Can you work these out from the drawing? Everything is in mm from the part's minimum corner. A direction names the side the tool comes from. Give positions to 0.01 mm unless a question says otherwise; leave off trailing zeros. Loops run counter-clockwise (first coordinate to the right, second up) from the corner with the lowest first, then second, coordinate; pieces in that order, holes last. Notation, with made-up numbers: (-12, 76) - (27, 76) arc R22 ccw to (27, 99) - close; hole circle Ø4 at (33, -39). An arc over 180 degrees is marked (long way). Answer in a Markdown table with one row per item.
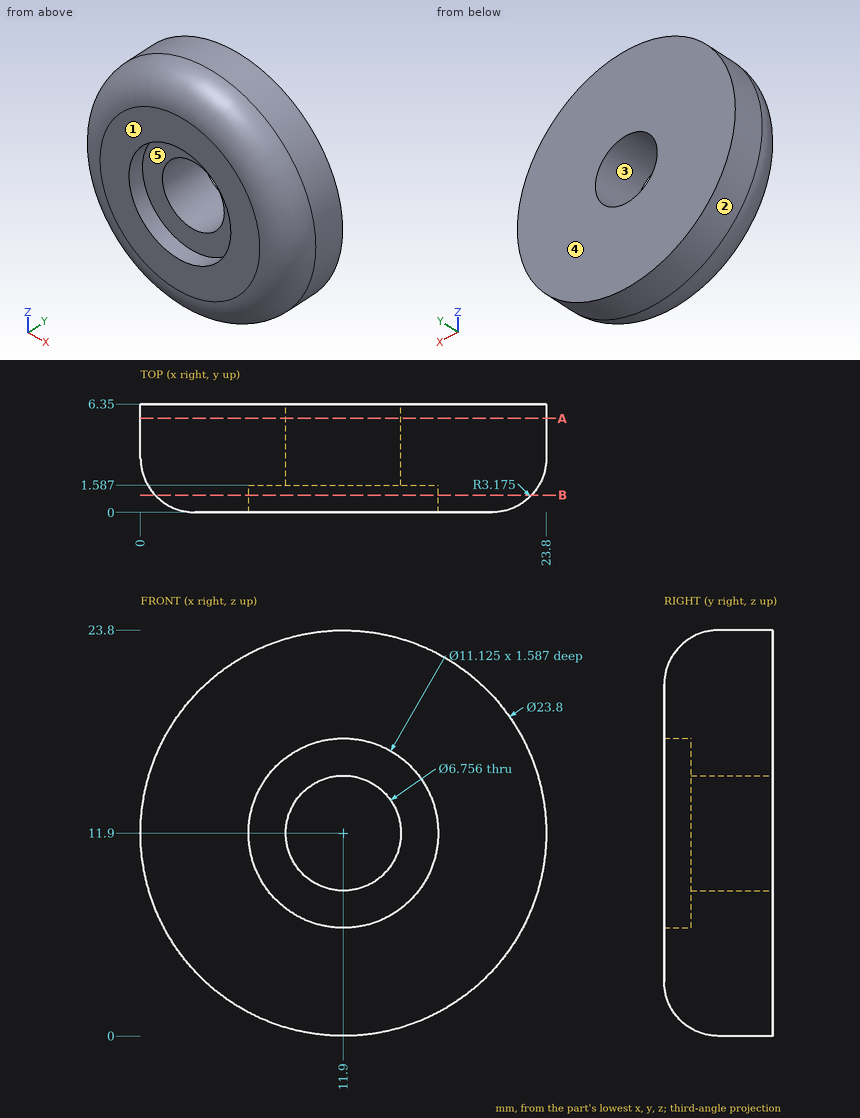
Q1. For pin 1 (1 mm diameter, centred on x = 15, z = 14, fed in from -Y); pin 2 (1.5 mm diameter, centred on y = 1, z = 12.5, fed in from +X); pin 3 (2 mm diameter, centred on y = 3.5, z = 6, fed in from -X) (1 decimal), each with a flat end and sliding along its axis, tell me the tip position at first contact or that it passes through.
Checked values:
| item | result |
|---|---|
| pin 1 | stops at y = 1.59 |
| pin 2 | stops at x = 23.45 |
| pin 3 | stops at x = 1.1 |
Q2. If I drill on line 1 (Z direction, x = 9.25, y = 0.5) (1 decimal); line 2 (Z direction, x = 14.25, y = 4.75) (1 decimal); line 3 (Y direction, x = 9.5, z = 16.5), over which ranges is the centre line in solid material (lowest first)? Write a range as [from, to].
Checked values:
| item | result |
|---|---|
| line 1 | z = [1.8, 7], [16.8, 22] |
| line 2 | z = [0.2, 9.5], [14.3, 23.6] |
| line 3 | y = [1.59, 6.35] |
Q3. On a 3-axis mill with a long thin cutter (end or side, diameter ignored), from which of +Z, -Z, +X, -X, +Y, -Y can I reach the whole of each face in a straight line? I mean the marked faces 4 and 5. Say none if no direction works.
Checked values:
| item | result |
|---|---|
| face 4 | +Z, -Z, +X, -X, +Y |
| face 5 | -Y |
Q4. Imagine slicing it at B-B, the plane y = 1. Write out the boundary of the cut face in (x, z) (1 decimal).
Checked values:
| item | result |
|---|---|
| outline | circle Ø22.1 at (11.9, 11.9); hole circle Ø11.1 at (11.9, 11.9) |
Q5. Imagine slicing it at A-A, the plane y = 5.5. Write out the boundary of the cut face in (x, z), and give its area (3 significant figures).
Checked values:
| item | result |
|---|---|
| outline | circle Ø23.8 at (11.9, 11.9); hole circle Ø6.76 at (11.9, 11.9) |
| area | 409 mm² |
Q6. If we mould it in two halves opening along Z, with no side actions, what happens to the marked faces 1, 2 and 3? For each: released by +Z, released by -Z, zero draft, split by the parting line, or undercut.
Checked values:
| item | result |
|---|---|
| face 1 | zero draft |
| face 2 | split by the parting line |
| face 3 | undercut |
